```python
from build123d import *

# Parameters (mm, degrees)
SKETCH_1_R          = 3.5
EXTRUDE_1_DEPTH     = 20
SKETCH_2_R          = 4.25
CUT_EXTRUDE_1_DEPTH = 20
SKETCH_3_R          = 4.25
CUT_EXTRUDE_2_DEPTH = 20


with BuildPart() as part:
    # 草图1 → 凸台-拉伸1 (new, symmetric)
    with BuildSketch(Plane.XY):
        Polygon((0, 0), (56.568542495, 56.568542495), (62.225396744, 50.911688245), (48.470353518, 37.156645019), (60.547431318, 8), (80, 8), (80, 0), align=None)
        with Locations((22.184677187, 9.156473773)):
            Circle(SKETCH_1_R, mode=Mode.SUBTRACT)
        Polygon((12.071067812, 5), (15.847671377, 8.776603565), (17.411991793, 5), align=None, mode=Mode.SUBTRACT)
        with BuildLine():
            Line((22.539170943, 15.468103131), (44.931612237, 37.860544425))
            Line((44.931612237, 37.860544425), (58.542895405, 5))
            Line((58.542895405, 5), (26.941798117, 5))
            ThreePointArc((26.941798117, 5), (26.493271042, 5.27903968), (26.545371373, 5.804706148))
            ThreePointArc((26.545371373, 5.804706148), (27.253512915, 11.291164467), (22.833720405, 14.61804341))
            ThreePointArc((22.833720405, 14.61804341), (22.420282519, 14.950846558), (22.539170943, 15.468103131))
        make_face(mode=Mode.SUBTRACT)
    extrude(amount=EXTRUDE_1_DEPTH, both=True)

    # 草图2 → 切除-拉伸1 (cut)
    with BuildSketch(Plane(origin=(0, 0, 0), x_dir=(0, 0, 1), z_dir=(-0.7071067811865488, 0.7071067811865464, 0))):
        with Locations(Location((0, 70, 0), (0, 0, 270))):
            Circle(SKETCH_2_R)
    extrude(amount=-CUT_EXTRUDE_1_DEPTH, mode=Mode.SUBTRACT)

    # 草图3 → 切除-拉伸2 (cut)
    with BuildSketch(Plane.XZ):
        with Locations(Location((70, 0, 0), (0, 0, 270))):
            Circle(SKETCH_3_R)
    extrude(amount=-CUT_EXTRUDE_2_DEPTH, mode=Mode.SUBTRACT)


solid = part.part
```
Input: part model. Units: mm. Frame: model coordinates. A direction names the side the tool comes from. Give positions to 0.01 mm unless a question says otherwise; leave off trailing zeros. Order: outer loops, then holes, each group sorted by start corner. A loop starts at its lowest first (then second) coordinate and runs counter-clockwise, first axis right, second up. Notation, with made-up numbers: M -3,16 L 1,16 A20 ccw 1,24 Z; hole C -24,0 d11. An arc over 180 degrees is marked long. One line per question, with ' | ' between items. Start each with the question number.
1. Section query C-C (y = 16.5). Return the cut outline in (x, z).
2. Pull-direction query (X, two-part tool) for faces 4 (the face through (52, 24, -20)), 5 (the face through (43, 5, 0)), 6 (the face through (54.424, 22.782, 0.28)); classes: released by +X, released by -X, zero draft, split by the parting line, or undercut.
3. First-contact query: pin 1 Ø1 at (x, z) = (67.5, 3) entering from +Y; pin 2 Ø8 at (y, z) = (18, 4) entering from -X; pin 3 Ø1.6 at (x, z) = (15.5, 3) entering from +Y. Flat tips, straight axial feed; report the tip coordinate or a pass-through.
4. Section query B-B (z = 0). Return the cut outline in (x, y).
5. Material intervals for probe 1 along Y at (x, z) = (53, 16); probe 2 along Y at (x, z) = (56, 12); probe 3 along X at (y, z) = (11, 0.5), sorted ascending. Write a range as [from, to].
6. Section query A-A (x = 70). Return the cut outline in (y, z), and give its area (3 significant figures).
7. Section query D-D (z = 6). Return the cut outline in (x, y), and give its area (3 significant figures).
8. Access query for faces 1 (the face through (58.501, 47.187, 0.28)), 2 (the face through (51.64, 21.66, 0.28)), 3 (the face through (41, 0, 0)). Directions: +Z, -Z, +X, -X, +Y, -Y. A direction counts if a zero-diameter tool reaches every point of the face in a straight line with its end or side. Return the directions, or none.
Here are the results:
1) outline: M 16.5,-20 L 23.57,-20 L 23.57,20 L 16.5,20 Z; M 53.78,-20 L 57.03,-20 L 57.03,20 L 53.78,20 Z
2) face 4: zero draft | face 5: undercut | face 6: released by +X
3) pin 1: y = 8 | pin 2: x = 14 | pin 3: y = 16.3
4) outline: M 0,0 L 65.75,0 L 65.75,8 L 60.55,8 L 48.47,37.16 L 52.15,40.84 L 46.49,46.49 Z; M 52.5,52.5 L 58.16,46.85 L 62.23,50.91 L 56.57,56.57 Z; M 74.25,0 L 80,0 L 80,8 L 74.25,8 Z; hole M 12.07,5 L 17.41,5 L 15.85,8.78 Z; hole C 22.18,9.16 d7; hole M 22.54,15.47 A0.5 ccw 22.83,14.62 A5.5 cw 26.55,5.8 A0.5 ccw 26.94,5 L 58.54,5 L 44.93,37.86 Z
5) probe 1: [0, 5], [18.38, 26.22], [41.69, 53] | probe 2: [0, 5], [11.14, 18.98], [44.69, 56] | probe 3: [11, 19.21], [25.16, 27.37], [56.06, 59.3]
6) outline: M 0,-20 L 8,-20 L 8,-4.25 L 0,-4.25 Z; M 0,4.25 L 8,4.25 L 8,20 L 0,20 Z | area: 252 mm²
7) outline: M 0,0 L 80,0 L 80,8 L 60.55,8 L 48.47,37.16 L 62.23,50.91 L 56.57,56.57 Z; hole M 12.07,5 L 17.41,5 L 15.85,8.78 Z; hole C 22.18,9.16 d7; hole M 22.54,15.47 A0.5 ccw 22.83,14.62 A5.5 cw 26.55,5.8 A0.5 ccw 26.94,5 L 58.54,5 L 44.93,37.86 Z | area: 1,010 mm²
8) face 1: +Z, -Z, +X | face 2: +Z, -Z | face 3: +Z, -Z, +X, -X, -Y
